The model under review builds one solid part; all positions refer to its coordinate system, in mm. A direction names the side the tool comes from. Give positions to 0.01 mm unless a question says otherwise; leave off trailing zeros. Loops run counter-clockwise (first coordinate to the right, second up) from the corner with the lowest first, then second, coordinate; pieces in that order, holes last. Notation, with made-up numbers: (-37.5, 40) - (-12.5, 40) arc R16 cw to (-12.5, 53) - close; hole circle Ø3 at (42, -12). An arc over 180 degrees is marked (long way). Return JSON: item names as keys, results as strings. Group by question number.
```python
from build123d import *

# Parameters (mm, degrees)
SKETCH1_R           = 5.08
SKETCH1_R_2         = 3.81
SKETCH1_R_3         = 2.286
BOSS_EXTRUDE1_DEPTH = 2.54
SKETCH2_R           = 1.524
BOSS_EXTRUDE2_DEPTH = 1.27
SKETCH3_R           = 2.286
BOSS_EXTRUDE3_DEPTH = 0.508
SCALE1_SCALE        = 1.5
CUT_EXTRUDE1_START  = 7.112
SKETCH4_R           = 1.5875
CUT_EXTRUDE1_DEPTH  = 10
SKETCH5_R           = 0.762
CUT_EXTRUDE2_DEPTH  = 22.655627009


with BuildPart() as part:
    # Sketch1 → Boss-Extrude1 (new body)
    # profile 1 of 3: a face of its own
    with BuildSketch(Plane.XY):
        Circle(SKETCH1_R)
        Circle(SKETCH1_R_2, mode=Mode.SUBTRACT)
    # profile 2 of 3: a face of its own
    with BuildSketch(Plane.XY):
        with BuildLine():
            ThreePointArc((4.955539349, -1.1176), (0, -5.08), (-4.955539349, -1.1176))
            Line((-4.955539349, -1.1176), (-2.229992707, -13.20292))
            ThreePointArc((-2.229992707, -13.20292), (-0.253014497, -10.428044969), (2.286, -12.7))
            ThreePointArc((2.286, -12.7), (2.271955031, -12.953014497), (2.229992707, -13.20292))
            Line((2.229992707, -13.20292), (4.955539349, -1.1176))
        make_face()
    # profile 3 of 3: a face of its own
    with BuildSketch(Plane.XY):
        with Locations((0, -12.7)):
            Circle(SKETCH1_R_3)
    extrude(amount=BOSS_EXTRUDE1_DEPTH)

    # Sketch2 → Boss-Extrude2 (add)
    with BuildSketch(Plane.XY.offset(2.54)):
        with Locations((0, -12.7)):
            Circle(SKETCH2_R)
    extrude(amount=BOSS_EXTRUDE2_DEPTH)

    # Sketch3 → Boss-Extrude3 (add)
    with BuildSketch(Plane.XY.offset(3.81)):
        with Locations((0, -12.7)):
            Circle(SKETCH3_R)
    extrude(amount=BOSS_EXTRUDE3_DEPTH)


with BuildPart() as part_1:
    # Scale1: scaled about (0, -6.091225053, 1.422264494)
    add(part.part.scale(SCALE1_SCALE).moved(Location((0, 3.045612526, -0.711132247))))

    # Sketch4 → Cut-Extrude1 (cut)
    with BuildSketch(Plane(origin=(0, 0, 0), x_dir=(0, 0, -1), z_dir=(1, 0, 0)).offset(CUT_EXTRUDE1_START)):
        with Locations(Location((-1.193867753, 3.045612527, 0), (0, 0, 180))):
            Circle(SKETCH4_R)
    extrude(amount=CUT_EXTRUDE1_DEPTH, mode=Mode.SUBTRACT)

    # Sketch5 → Cut-Extrude2 (cut, through all)
    with BuildSketch(Plane(origin=(0, 0, 0), x_dir=(0, 0, -1), z_dir=(1, 0, 0))):
        with Locations((-1.193867753, 3.045612527)):
            Circle(SKETCH5_R)
    extrude(amount=CUT_EXTRUDE2_DEPTH, mode=Mode.SUBTRACT)


solid = part_1.part
```
1) We need section C-C, the plane x = 6.75. Write out the cut boundary in (y, z).
2) We need section A-A, the plane x = 0. Write out the cut boundary in (y, z), plus the area to 3 significant figures.
3) Tool access review of faces 4 (the face through (-5.418, -7.568, 1.167)), 5 (the face through (6.378, 3.274, 0.467)), 6 (the face through (-0.496, -18.236, 4.038)): name each direction out of +Z, -Z, +X, -X, +Y, -Y from which nothing blocks a thin tool from reaching the whole face with its end or side.
4) To check wall thickness, follow line 1 (X direction, y = 3, z = 2.5); line 2 (Z direction, x = -6, y = -4.5); line 3 (Y direction, x = -0.75, z = 2.25). State the ranges of each line that lie inside material, in increasing order.
5) Draft analysis for pull direction X (two halves, no side actions). For faces 1 (the face through (1.582, -19.047, 5.38)), 2 (the face through (3.072, 7.865, 1.167)), 3 (the face through (7.112, 4, 1)), state which applies: +X half, -X half, draft (parallel to the pull), parting line (faces both ways), or undercut.
6) For pin 1 Ø7.5 at (x, y) = (-0.5, -0.5) entering from +Z; pin 2 Ø1.5 at (x, z) = (-3.5, 5) entering from +Y; pin 3 Ø3 at (y, z) = (-8.5, 2) entering from +X, all flat-tipped, find the tip position at first contact; note any pin that passes through.
7) We need section B-B, the plane y = 6. Write out the cut boundary in (x, z), plus the area to 3 significant figures.
8) We need section D-D, the plane z = 1.25. Write out the cut boundary in (x, y) (3 decimals).
Findings:
{
 "1": {"outline": "(-1.66, -0.71) - (6.58, -0.71) - (6.58, 3.1) - (-1.66, 3.1) - close; hole circle Ø1.52 at (3.05, 1.19)"},
 "2": {"outline": "(-19.43, -0.71) - (-2.67, -0.71) - (-2.67, 3.1) - (-13.72, 3.1) - (-13.72, 5) - (-12.58, 5) - (-12.58, 5.77) - (-19.43, 5.77) - (-19.43, 5) - (-18.29, 5) - (-18.29, 3.1) - (-19.43, 3.1) - close; (8.76, -0.71) - (10.67, -0.71) - (10.67, 3.1) - (8.76, 3.1) - close", "area": "85.1 mm^2"},
 "3": {"face 4": "+Z, -Z, -X, -Y", "face 5": "+X", "face 6": "none"},
 "4": {"line 1": "x = -7.62 to -5.71, 5.71 to 7.11", "line 2": "z = -0.71 to 3.1", "line 3": "y = -19.35 to -2.62, 8.71 to 10.63"},
 "5": {"face 1": "parting line", "face 2": "undercut", "face 3": "+X half"},
 "6": {"pin 1": "stops at z = 3.1", "pin 2": "stops at y = -13.96", "pin 3": "stops at x = 5.55"},
 "7": {"outline": "(-7.02, -0.71) - (-4.89, -0.71) - (-4.89, 3.1) - (-7.02, 3.1) - close; (4.89, -0.71) - (7.02, -0.71) - (7.02, 3.1) - (4.89, 3.1) - close", "area": "16.2 mm^2"},
 "8": {"outline": "(-7.433, 1.369) - (-3.345, -16.759) arc R3.429 ccw to (3.345, -16.759) - (7.433, 1.369) arc R7.62 ccw to (7.453, 1.459) - (7.112, 1.459) - (7.112, 2.286) - (5.664, 2.286) arc R5.715 cw (long way) to (5.664, 3.806) - (7.112, 3.806) - (7.112, 4.632) - (7.453, 4.632) arc R7.62 ccw (long way) to start"}
}
